```python
from build123d import *

# Parameters (mm, degrees)
SKETCH_1_W          = 10
SKETCH_1_H          = 3
SKETCH_1_W_2        = 6
EXTRUDE_1_DEPTH     = 5
SKETCH_2_R          = 1.6
CUT_EXTRUDE_1_DEPTH = 10
CHAMFER_1_SIZE      = 2


with BuildPart() as part:
    # 草图1 → 凸台-拉伸1 (new, symmetric)
    with BuildSketch(Plane.XY):
        Rectangle(SKETCH_1_W, SKETCH_1_H)
        with Locations((0, 1.5)):
            Rectangle(SKETCH_1_W_2, SKETCH_1_H)
    extrude(amount=EXTRUDE_1_DEPTH, both=True)

    # 草图2 → 切除-拉伸1 (cut)
    with BuildSketch(Plane(origin=(0, 3, 0), x_dir=(1, 0, 0), z_dir=(0, 1, 0))):
        with Locations(Location((0, 0, 0), (0, 0, 270))):
            Circle(SKETCH_2_R)
    extrude(amount=-CUT_EXTRUDE_1_DEPTH, mode=Mode.SUBTRACT)

    # 倒角1
    chamfer_1_edges = [part.edges().sort_by_distance(p)[0] for p in [
        (5, -1.5, 0),
        (-5, -1.5, 0),
    ]]
    chamfer(chamfer_1_edges, length=CHAMFER_1_SIZE)


solid = part.part
```
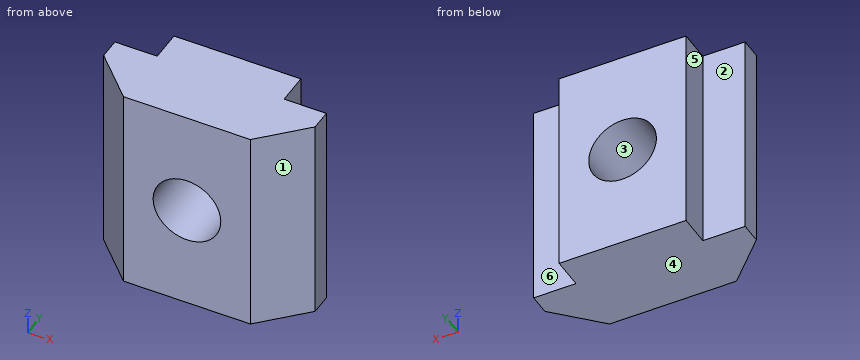
The listing builds one solid part. Answer for the finished solid, in the listing's coordinates (mm). Face numbers are marked on the shaded views. A direction names the side the tool comes from. Coordinates: 2 decimals unless noted, no trailing zeros. Write each loop counter-clockwise with the first axis right and the second up, starting at its lowest first coordinate (ties: lowest second). Pieces come first, ordered by that corner, then holes. Notation, with made-up numbers: M 52,5 L 63,5 A23 cw 63,15 Z; hole C 86,-0.75 d4. An arc over 180 degrees is marked long. Use a Markdown table: item, result. Add a question column.
1. Section D-D (z = -4.25) is taken. Give the vertices of the cut face in (x, y).
2. Given P1, Ø2, axis at y = 2, z = 4, coming from the -X side; P2, Ø0.8, axis at y = 2.5, z = 2.5, coming from the +X side, each flat-ended and moving along its own axis, determine where each tip first touches the part or whether it passes through.
3. For a pull along X with two mould halves and no side action, classify the marked faces 1, 2 and 3 as +X half, -X half, draft (parallel to the pull), parting line (faces both ways), or undercut.
4. Which of the six approach directions +Z, -Z, +X, -X, +Y, -Y give full straight-line access (tool end or side, diameter ignored) to the marked faces 4, 5 and 6?
5. Section C-C (y = -0.9) is taken. Give the vertices of the cut face in (x, z), plus the area to 3 significant figures.
6. Section B-B (x = 0) is taken. Give the vertices of the cut face in (y, z).
7. Section A-A (z = 0) is taken. Give the vertices of the cut face in (x, y).
8. Straight lines are drawn through the part: line 1 along X through (y, z) = (0.9, 0); line 2 along X through (y, z) = (-0.35, 0); line 3 along X through (y, z) = (2, -2.25). For each, find the intervals that lie inside material, in ascending order. Write a range as [from, to].
Data:
| question | item | result |
|---|---|---|
| 1 | outline | M -5,0.5 L -3,-1.5 L 3,-1.5 L 5,0.5 L 5,1.5 L 3,1.5 L 3,3 L -3,3 L -3,1.5 L -5,1.5 Z |
| 2 | P1 | stops at x = -5 |
| 2 | P2 | stops at x = 3 |
| 3 | face 1 | +X half |
| 3 | face 2 | draft |
| 3 | face 3 | undercut |
| 4 | face 4 | -Z, +X, -X, +Y, -Y |
| 4 | face 5 | +Z, -Z, -X, +Y |
| 4 | face 6 | +Z, -Z, +X, +Y |
| 5 | outline | M -3.6,-5 L 3.6,-5 L 3.6,5 L -3.6,5 Z; hole C 0,0 d3.2 |
| 5 | area | 64.0 mm2 |
| 6 | outline | M -1.5,-5 L 3,-5 L 3,-1.6 L -1.5,-1.6 Z; M -1.5,1.6 L 3,1.6 L 3,5 L -1.5,5 Z |
| 7 | outline | M -5,0.5 L -3,-1.5 L -1.6,-1.5 L -1.6,3 L -3,3 L -3,1.5 L -5,1.5 Z; M 1.6,-1.5 L 3,-1.5 L 5,0.5 L 5,1.5 L 3,1.5 L 3,3 L 1.6,3 Z |
| 8 | line 1 | x = [-5, -1.6], [1.6, 5] |
| 8 | line 2 | x = [-4.15, -1.6], [1.6, 4.15] |
| 8 | line 3 | x = [-3, 3] |
